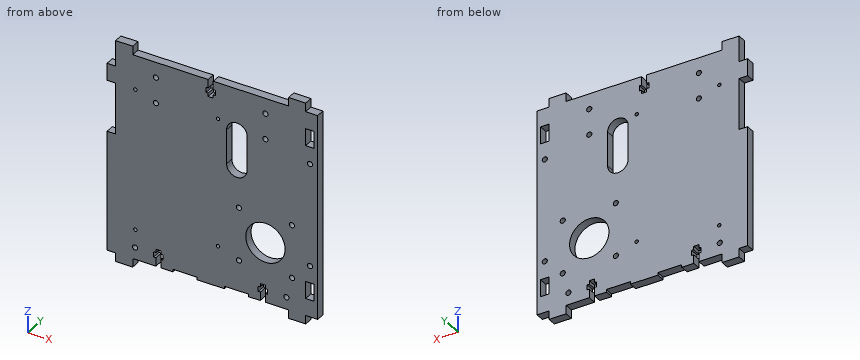
from build123d import *

# Parameters (mm, degrees)
SKETCH2_W           = 121
SKETCH2_H           = 120
SKETCH2_R           = 11.5
SKETCH2_R_2         = 1.5
SKETCH2_R_3         = 1
BOSS_EXTRUDE1_DEPTH = 5
SKETCH3_W           = 10
SKETCH3_H           = 5
SKETCH3_W_2         = 2
SKETCH3_H_2         = 120
BOSS_EXTRUDE2_DEPTH = 5
SKETCH4_R           = 1.5
SKETCH4_W           = 5
SKETCH4_H           = 10
SKETCH4_H_2         = 30
SKETCH4_W_2         = 14
SKETCH4_H_3         = 1.5
CUT_EXTRUDE1_DEPTH  = 175.043098111


with BuildPart() as part:
    # Sketch2 → Boss-Extrude1 (new body)
    with BuildSketch(Plane(origin=(0, 0, 0), x_dir=(1, 0, 0), z_dir=(0, 1, 0))):
        with Locations((-60.5, 60)):
            Rectangle(SKETCH2_W, SKETCH2_H)
        with Locations(Location((-28.5, 85, 0), (0, 0, 270))):
            Circle(SKETCH2_R, mode=Mode.SUBTRACT)
        with Locations(Location((-44, 100.5, 0), (0, 0, 270))):
            Circle(SKETCH2_R_2, mode=Mode.SUBTRACT)
        with Locations(Location((-13, 100.5, 0), (0, 0, 270))):
            Circle(SKETCH2_R_2, mode=Mode.SUBTRACT)
        with Locations(Location((-13, 69.5, 0), (0, 0, 270))):
            Circle(SKETCH2_R_2, mode=Mode.SUBTRACT)
        with Locations(Location((-44, 69.5, 0), (0, 0, 270))):
            Circle(SKETCH2_R_2, mode=Mode.SUBTRACT)
        with Locations(Location((-92.5, 24, 0), (0, 0, 270))):
            Circle(SKETCH2_R_2, mode=Mode.SUBTRACT)
        with Locations(Location((-92.5, 9, 0), (0, 0, 270))):
            Circle(SKETCH2_R_2, mode=Mode.SUBTRACT)
        with Locations(Location((-28.5, 9, 0), (0, 0, 90))):
            Circle(SKETCH2_R_2, mode=Mode.SUBTRACT)
        with Locations(Location((-28.5, 24, 0), (0, 0, 90))):
            Circle(SKETCH2_R_2, mode=Mode.SUBTRACT)
        with Locations(Location((-104.46, 19.97, 0), (0, 0, 270))):
            Circle(SKETCH2_R_3, mode=Mode.SUBTRACT)
        with Locations(Location((-104.46, 102.52, 0), (0, 0, 270))):
            Circle(SKETCH2_R_3, mode=Mode.SUBTRACT)
        with Locations(Location((-56.2, 96.17, 0), (0, 0, 270))):
            Circle(SKETCH2_R_3, mode=Mode.SUBTRACT)
        with Locations(Location((-56.2, 21.24, 0), (0, 0, 270))):
            Circle(SKETCH2_R_3, mode=Mode.SUBTRACT)
    extrude(amount=BOSS_EXTRUDE1_DEPTH)

    # Sketch3 → Boss-Extrude2 (add)
    with BuildSketch(Plane(origin=(0, 5, 0), x_dir=(1, 0, 0), z_dir=(0, 1, 0))):
        with Locations((-111, 122.5)):
            Rectangle(SKETCH3_W, SKETCH3_H)
        with Locations((-10, 122.5)):
            Rectangle(SKETCH3_W, SKETCH3_H)
        with Locations((-10, -2.5)):
            Rectangle(SKETCH3_W, SKETCH3_H)
        with Locations((-111, -2.5)):
            Rectangle(SKETCH3_W, SKETCH3_H)
        with Locations((1, 60)):
            Rectangle(SKETCH3_W_2, SKETCH3_H_2)
    extrude(amount=-BOSS_EXTRUDE2_DEPTH)

    # Sketch4 → Cut-Extrude1 (cut, through all)
    with BuildSketch(Plane(origin=(0, 5, 0), x_dir=(1, 0, 0), z_dir=(0, 1, 0))):
        with Locations(Location((-2.5, 90, 0), (0, 0, 270))):
            Circle(SKETCH4_R)
        with Locations(Location((-2.5, 30, 0), (0, 0, 90))):
            Circle(SKETCH4_R)
        with Locations(Location((-16.3, 113, 0), (0, 0, 270))):
            Circle(SKETCH4_R)
        with Locations(Location((-104.7, 113, 0), (0, 0, 90))):
            Circle(SKETCH4_R)
        with Locations((-2.5, 105)):
            Rectangle(SKETCH4_W, SKETCH4_H)
        with Locations((-2.5, 15)):
            Rectangle(SKETCH4_W, SKETCH4_H)
        with Locations((-118.5, 35)):
            Rectangle(SKETCH4_W, SKETCH4_H_2)
        with Locations((-118.5, 5)):
            Rectangle(SKETCH4_W, SKETCH4_H)
        with Locations((-75.5, 119.25)):
            Rectangle(SKETCH4_W_2, SKETCH4_H_3)
        with Locations((-45.5, 119.25)):
            Rectangle(SKETCH4_W_2, SKETCH4_H_3)
        Polygon((-31.5, 120), (-31.5, 115), (-32.75, 115), (-32.75, 112), (-31.5, 112), (-31.5, 110), (-28.5, 110), (-28.5, 112), (-27.25, 112), (-27.25, 115), (-28.5, 115), (-28.5, 120), align=None)
        Polygon((-92.5, 120), (-89.5, 120), (-89.5, 115), (-88.25, 115), (-88.25, 112), (-89.5, 112), (-89.5, 110), (-92.5, 110), (-92.5, 112), (-93.75, 112), (-93.75, 115), (-92.5, 115), align=None)
        with BuildLine():
            Line((-51.2, 26), (-51.2, 46))
            ThreePointArc((-51.2, 46), (-45.2, 52), (-39.2, 46))
            Line((-39.2, 46), (-39.2, 26))
            ThreePointArc((-39.2, 26), (-45.2, 20), (-51.2, 26))
        make_face()
        Polygon((-62, 0), (-62, 5), (-63.25, 5), (-63.25, 8), (-62, 8), (-62, 10), (-59, 10), (-59, 8), (-57.75, 8), (-57.75, 5), (-59, 5), (-59, 0), align=None)
    extrude(amount=-CUT_EXTRUDE1_DEPTH, mode=Mode.SUBTRACT)


solid = part.part
Model file for the job. Use its own axes, mm. Round coordinates to 2 decimals unless told otherwise and drop trailing zeros. Order: outer loops, then holes, each group sorted by start corner. A loop starts at its lowest first (then second) coordinate and runs counter-clockwise, first axis right, second up.
(1) Band-saw the part on B-B (x = -48.5). List the corners of the cut face in (y, z), then the cut area to 3 significant figures.
(2) Pin check, flat tips, straight feed: pin 1 (2.5 mm diameter, centred on y = 2, z = 1.5, fed in from -X); pin 2 (1.4 mm diameter, centred on x = -32, y = 2.5, fed in from +Z); pin 3 (0.9 mm diameter, centred on x = -60.5, y = 2, fed in from +Z). Stop position of each tip, or through.
(3) Band-saw the part on A-A (x = -13). List the corners of the cut face in (y, z).
(4) Drill centre lines: line 1 (X direction, y = 3.45, z = -113); line 2 (X direction, y = 2.5, z = -109); line 3 (X direction, y = 1.85, z = -1.5). Where is each one in solid material? Low to high.
(5) Band-saw the part on C-C (z = -90). List the corners of the cut face in (x, y), then the cut area to 3 significant figures.
(6) Band-saw the part on D-D (y = 3.55). Give the number of separate pieces and of enclosed holes in the cut face, then the cut area to 3 significant figures.
Verdict:
1. outline: (0, -118.5) - (5, -118.5) - (5, -51.01) - (0, -51.01) - close; (0, -20.99) - (5, -20.99) - (5, 0) - (0, 0) - close
1. area: 442 mm2
2. pin 1: stops at x = -116
2. pin 2: stops at z = 0
2. pin 3: stops at z = -10
3. outline: (0, -125) - (5, -125) - (5, -102) - (0, -102) - close; (0, -99) - (5, -99) - (5, -71) - (0, -71) - close; (0, -68) - (5, -68) - (5, 5) - (0, 5) - close
4. line 1: x = -121 to -106.2, -103.2 to -93.75, -88.25 to -32.75, -27.25 to -17.8, -14.8 to 2
4. line 2: x = -121 to -5, 0 to 2
4. line 3: x = -116 to -62, -59 to 2
5. outline: (-121, 0) - (-38.86, 0) - (-38.86, 5) - (-121, 5) - close; (-18.14, 0) - (-4, 0) - (-4, 5) - (-18.14, 5) - close; (-1, 0) - (2, 0) - (2, 5) - (-1, 5) - close
5. area: 496 mm2
6. separate pieces: 1
6. enclosed holes: 20
6. area: 13,600 mm2
